Model file for the job. Use its own axes, mm. A direction names the side the tool comes from. Coordinates: 2 decimals unless noted, no trailing zeros. Write each loop counter-clockwise with the first axis right and the second up, starting at its lowest first coordinate (ties: lowest second). Pieces come first, ordered by that corner, then holes.
Q1. Pin check, flat tips, straight feed: P1, Ø1, axis at y = 4, z = -12, coming from the -X side; P2, Ø10, axis at y = 10, z = -3, coming from the +X side; P3, Ø11.5, axis at x = 11, z = 2, coming from the +Y side; P4, Ø8, axis at x = 5, z = 9, coming from the +Y side. Stop position of each tip, or through.
Q2. Pull direction Z, two halves, no side cores. Call faces 1 (the flat face through (6, 9, -25.4)), 2 (the flat face through (0, 15, 0)), 3 (the flat face through (7, 10, 22.4)): released by +Z, released by -Z, zero draft, split by the parting line, or undercut.
Q3. Which spindle directions (+Z, -Z, +X, -X, +Y, -Y) get a long thin tool onto all of the face, cutting with end or side? Do faces 4 (the flat face through (11, 2, 12.25)), 5 (the flat face through (6, 9, 25.4)), 6 (the flat face through (10, 4, 0)). Say none if no direction does.
Q4. Band-saw the part on A-A, the plane z = 15. Write the cut outline in (x, y), plus the area to 3 significant figures.
Q5. Band-saw the part on C-C, the plane y = 2. Write the cut outline in (x, z).
Q6. Band-saw the part on B-B, the plane x = 11. Write the cut outline in (y, z).
Q7. Band-saw the part on D-D, the plane y = 18. Write the cut outline in (x, z), plus the area to 3 significant figures.
Q8. Drill centre lines: probe 1 along Z at (x, y) = (14, 3.5); probe 2 along Z at (x, y) = (5.75, 8.75); probe 3 along Z at (x, y) = (8.25, 2.75). Where is each one in solid material? Low to high.
from build123d import *

# Parameters (mm, degrees)
BOSS_EXTRUDE1_DEPTH      = 25.4
SKETCH3_W                = 17
SKETCH3_H                = 44.8
CUT_EXTRUDE1_DEPTH       = 26
M5_CLEARANCE_SLOT1_DEPTH = 4


# Read off the part's stored shape, not the designer's step: M5 Clearance Slot1
with BuildPart() as part:
    # Sketch2 → Boss-Extrude1 (new, symmetric)
    with BuildSketch(Plane.XY):
        Polygon((0, 0), (0, 30), (20, 0), align=None)
    extrude(amount=BOSS_EXTRUDE1_DEPTH, both=True)

    # Sketch3 → Cut-Extrude1 (cut)
    with BuildSketch(Plane(origin=(0, 30, 0), x_dir=(1, 0, 0), z_dir=(0, 1, 0))):
        with Locations((11.5, 0)):
            Rectangle(SKETCH3_W, SKETCH3_H)
    extrude(amount=-CUT_EXTRUDE1_DEPTH, mode=Mode.SUBTRACT)

    # M5 Clearance Slot1 outline → M5 Clearance Slot1 (cut)
    with BuildSketch(Plane(origin=(0, 0, 0), x_dir=(1, 0, 0), z_dir=(0, 1, 0))):
        with BuildLine():
            Line((9, 12.25), (12, 12.25))
            ThreePointArc((12, 12.25), (14.75, 15), (12, 17.75))
            Line((12, 17.75), (9, 17.75))
            ThreePointArc((9, 17.75), (6.25, 15), (9, 12.25))
        make_face()
        with BuildLine():
            Line((9, -17.75), (12, -17.75))
            ThreePointArc((12, -17.75), (14.75, -15), (12, -12.25))
            Line((12, -12.25), (9, -12.25))
            ThreePointArc((9, -12.25), (6.25, -15), (9, -17.75))
        make_face()
    extrude(amount=M5_CLEARANCE_SLOT1_DEPTH, mode=Mode.SUBTRACT)


solid = part.part
Answer sheet:
1. P1: stops at x = 0
1. P2: stops at x = 3
1. P3: stops at y = 4
1. P4: stops at y = 28.5
2. face 1: released by -Z
2. face 2: zero draft
2. face 3: undercut
3. face 4: +Y, -Y
3. face 5: +Z, +X, -X, +Y, -Y
3. face 6: +X, +Y
4. outline: (0, 0) - (6.25, 0) - (6.25, 4) - (3, 4) - (3, 25.5) - (0, 30) - close; (14.75, 0) - (20, 0) - (17.33, 4) - (14.75, 4) - close
4. area: 112 mm2
5. outline: (0, -25.4) - (18.67, -25.4) - (18.67, 25.4) - (0, 25.4) - close; hole (9, -17.75) - (12, -17.75) arc R2.75 ccw to (12, -12.25) - (9, -12.25) arc R2.75 ccw to start; hole (9, 12.25) - (12, 12.25) arc R2.75 ccw to (12, 17.75) - (9, 17.75) arc R2.75 ccw to start
6. outline: (0, -25.4) - (13.5, -25.4) - (13.5, -22.4) - (4, -22.4) - (4, -17.75) - (0, -17.75) - close; (0, -12.25) - (4, -12.25) - (4, 12.25) - (0, 12.25) - close; (0, 17.75) - (4, 17.75) - (4, 22.4) - (13.5, 22.4) - (13.5, 25.4) - (0, 25.4) - close
7. outline: (0, -25.4) - (8, -25.4) - (8, -22.4) - (3, -22.4) - (3, 22.4) - (8, 22.4) - (8, 25.4) - (0, 25.4) - close
7. area: 182 mm2
8. probe 1: z = -25.4 to -16.89, -13.11 to 13.11, 16.89 to 25.4
8. probe 2: z = -25.4 to -22.4, 22.4 to 25.4
8. probe 3: z = -25.4 to -17.65, -12.35 to 12.35, 17.65 to 25.4
